Source: three-view drawing plus pictorial views. Frame: mm from the lowest corner of the part. A direction names the side the tool comes from. Round coordinates to 2 decimals unless told otherwise and drop trailing zeros. Write each loop counter-clockwise with the first axis right and the second up, starting at its lowest first coordinate (ties: lowest second). Pieces come first, ordered by that corner, then holes. Notation, with made-up numbers: M -12.5,-19.75 L 4.5,-19.75 A21 ccw 4.5,-8.75 Z; hole C 61,56.25 d4. An arc over 180 degrees is marked long. Answer in a Markdown table with one row per item.
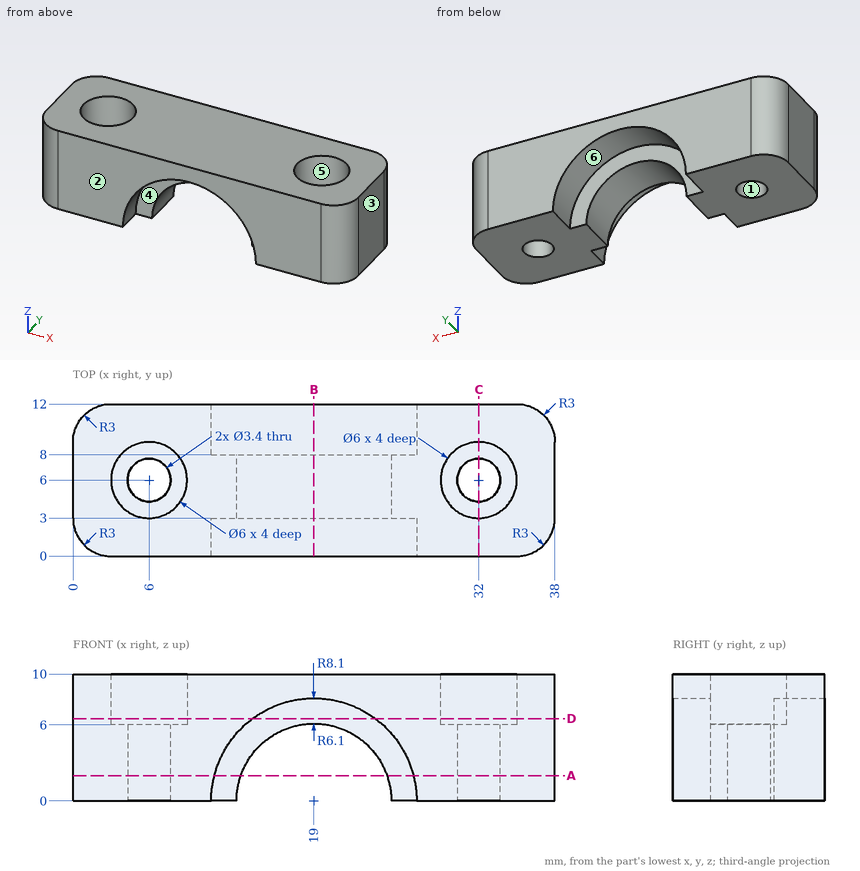
Q1. Section D-D (z = 6.5). Return loops of the section in (x, y).
Solutions:
| item | result |
|---|---|
| outline | M 0,3 A3 ccw 3,0 L 14.17,0 L 14.17,3 L 23.83,3 L 23.83,0 L 35,0 A3 ccw 38,3 L 38,9 A3 ccw 35,12 L 23.83,12 L 23.83,8 L 14.17,8 L 14.17,12 L 3,12 A3 ccw 0,9 Z; hole C 6,6 d6; hole C 32,6 d6 |
Q2. Contact query for flat-ended pins moving along their axis: pin 1 Ø2 at (x, z) = (16, 3) entering from +Y; pin 2 Ø3.5 at (x, y) = (32, 6) entering from +Z. Output: stop coordinate, or through.
Solutions:
| item | result |
|---|---|
| pin 1 | passes through |
| pin 2 | stops at z = 6 |
Q3. Access query for the marked faces 4, 5 and 6. Directions: +Z, -Z, +X, -X, +Y, -Y. A direction counts if a zero-diameter tool reaches every point of the face in a straight line with its end or side. Return the directions, or none.
Solutions:
| item | result |
|---|---|
| face 4 | -Z, -Y |
| face 5 | +Z |
| face 6 | -Z, +Y |
Q4. Section B-B (x = 19). Return loops of the section in (y, z), and give its area (3 significant figures).
Solutions:
| item | result |
|---|---|
| outline | M 0,8.1 L 3,8.1 L 3,6.1 L 8,6.1 L 8,8.1 L 12,8.1 L 12,10 L 0,10 Z |
| area | 32.8 mm2 |
Q5. Section C-C (x = 32). Return loops of the section in (y, z).
Solutions:
| item | result |
|---|---|
| outline | M 0,0 L 4.3,0 L 4.3,6 L 3,6 L 3,10 L 0,10 Z; M 7.7,0 L 12,0 L 12,10 L 9,10 L 9,6 L 7.7,6 Z |
Q6. Section A-A (z = 2). Return loops of the section in (x, y).
Solutions:
| item | result |
|---|---|
| outline | M 0,3 A3 ccw 3,0 L 11.15,0 L 11.15,3 L 13.24,3 L 13.24,8 L 11.15,8 L 11.15,12 L 3,12 A3 ccw 0,9 Z; M 24.76,3 L 26.85,3 L 26.85,0 L 35,0 A3 ccw 38,3 L 38,9 A3 ccw 35,12 L 26.85,12 L 26.85,8 L 24.76,8 Z; hole C 6,6 d3.4; hole C 32,6 d3.4 |
Q7. Pull-direction query (Y, two-part tool) for the marked faces 1, 2 and 3; classes: pulls with the +Y half, pulls with the -Y half, needs draft (parallel to the pull), parting line crosses it, or undercut.
Solutions:
| item | result |
|---|---|
| face 1 | undercut |
| face 2 | pulls with the -Y half |
| face 3 | needs draft |
Q8. Material intervals for probe 1 along X at (y, z) = (8.25, 7.5); probe 2 along Y at (x, z) = (6, 1.7); probe 3 along Y at (x, z) = (6, 7.65), sorted ascending.
Solutions:
| item | result |
|---|---|
| probe 1 | x = 0 to 4.02, 7.98 to 15.94, 22.06 to 30.02, 33.98 to 38 |
| probe 2 | y = 0 to 4.3, 7.7 to 12 |
| probe 3 | y = 0 to 3, 9 to 12 |
